Part model, mm, in its own coordinate system. Face numbers are marked on the shaded views. A direction names the side the tool comes from. Coordinates: 2 decimals unless noted, no trailing zeros. Write each loop counter-clockwise with the first axis right and the second up, starting at its lowest first coordinate (ties: lowest second). Pieces come first, ordered by that corner, then holes. Notation, with made-up numbers: M 16.25,-14 L 31.25,-14 A25 ccw 31.25,19 Z; hole C 29.5,-4 d2. An arc over 180 degrees is marked long. Use a Markdown table: item, result. Add a question column.
Q1. Tool access for the marked faces 1 and 2: list every direction of +Z, -Z, +X, -X, +Y, -Y with a clear straight run to the whole face (end or side of a thin tool).
Q2. Wall check: L1, parallel to X at y = -289, z = 15.25. Give the ranges that are in metal, low to high. Write a range as from..to.
Q3. Pin check, flat tips, straight feed: pin 1 Ø1.5 at (y, z) = (-326, 11) entering from +X; pin 2 Ø6 at (x, z) = (-319, 12) entering from -Y. Stop position of each tip, or through.
Q4. Slice it at C-C on x = -317. Write the cut outline in (y, z).
Q5. Slice it at A-A on z = 16.75. Write the cut outline in (x, y), then the cut area to 3 significant figures.
Q6. Slice it at B-B on y = -317. Write the cut outline in (x, z), then the cut area to 3 significant figures.
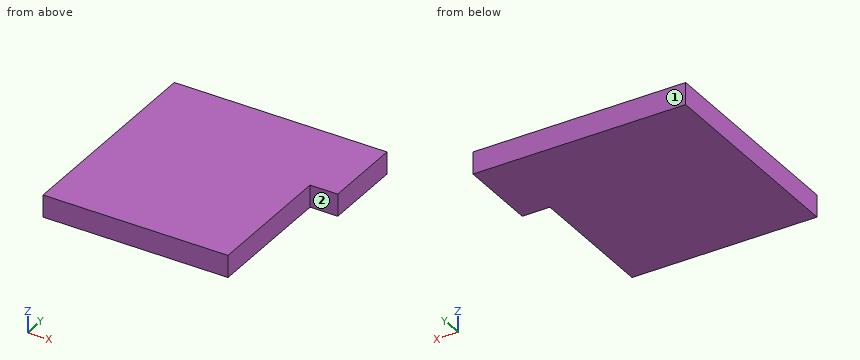
from build123d import *

# Parameters (mm, degrees)
F2_DEPTH  = 20
F3_W      = 217
F3_H      = 242
F3_W_2    = 167
F3_H_2    = 192
F4_DEPTH  = 240
F5_W      = 48
F5_H      = 72
F6_DEPTH  = 250
F7_W      = 79
F7_H      = 85
F8_DEPTH  = 25
F10_DEPTH = 25
F12_DEPTH = 240.001


with BuildPart() as f2:
    # F1 (on face) → F2 (new body)
    with BuildSketch(Plane.XY):
        Polygon((-497, -215), (-497, -231), (-497, -293), (-497, -407), (-330, -407), (-330, -287), (-330, -215), align=None)
    extrude(amount=F2_DEPTH)

    # F3 (on face) → F4 (join)
    with BuildSketch(Plane.XY):
        with Locations((-413.5, -311)):
            Rectangle(F3_W, F3_H)
        with Locations((-413.5, -311)):
            Rectangle(F3_W_2, F3_H_2, mode=Mode.SUBTRACT)
    extrude(amount=F4_DEPTH)

    # F5 (on face) → F6 (cut)
    with BuildSketch(Plane.XY.offset(20)):
        with Locations((-306, -251)):
            Rectangle(F5_W, F5_H)
    extrude(amount=F6_DEPTH, mode=Mode.SUBTRACT)

    # F7 (on face) → F8 (cut)
    with BuildSketch(Plane.YZ.offset(-497)):
        with Locations((-309.5, 177.5)):
            Rectangle(F7_W, F7_H)
    extrude(amount=-F8_DEPTH, mode=Mode.SUBTRACT)

    # F9 (on face) → F10 (join, through all)
    with BuildSketch(Plane.YZ.offset(-497)):
        Polygon((-270, 135), (-270, 220), (-290, 220), (-290, 155), (-349, 155), (-349, 135), align=None)
    extrude(amount=-F10_DEPTH)

    # F11 (on face) → F12 (cut, through all)
    with BuildSketch(Plane.XY.offset(240)):
        Polygon((-497, -407), (-497, -215), (-305, -215), (-305, -190), (-522, -190), (-522, -432), (-305, -432), (-305, -287), (-330, -287), (-330, -407), align=None)
    extrude(amount=-F12_DEPTH, mode=Mode.SUBTRACT)


solid = f2.part
Recorded:
| question | item | result |
|---|---|---|
| 1 | face 1 | +Z, -Z, +X, -X, +Y |
| 1 | face 2 | +Z, -Z, +X, -Y |
| 2 | L1 | -497..-330 |
| 3 | pin 1 | x = -330 |
| 3 | pin 2 | y = -287 |
| 4 | outline | M -287,0 L -215,0 L -215,20 L -287,20 Z |
| 5 | outline | M -497,-407 L -330,-407 L -330,-287 L -305,-287 L -305,-215 L -497,-215 Z |
| 5 | area | 33,900 mm² |
| 6 | outline | M -497,0 L -330,0 L -330,20 L -497,20 Z |
| 6 | area | 3,340 mm² |
